Verification items for the finished model (mm, model axes). A direction names the side the tool comes from. Coordinates: 2 decimals unless noted, no trailing zeros. Write each loop counter-clockwise with the first axis right and the second up, starting at its lowest first coordinate (ties: lowest second). Pieces come first, ordered by that corner, then holes. Notation, with made-up numbers: (-38, -1) -> (-18, -1) arc R20 cw to (-18, 33) -> close; hole circle Ø6 at (25.5, 58.25). An arc over 180 degrees is marked (long way). Answer in a Markdown table with one row per item.
```python
from build123d import *

# Parameters (mm, degrees)
F1_DEPTH = 3.302
F2_R     = 3.81
F3_R     = 2.54
F5_D     = 1.905
F6_R     = 1.27


with BuildPart() as f1:
    # F0 (on Top) → F1 (new body)
    with BuildSketch(Plane.XY):
        Polygon((2.54, 0), (0, 0), (0, -18.206947), (-8.938958, -15.811761), (-10.669027, -27.110069), (5.650751, -29.609057), (7.62, -24.926274), (7.62, -14.766274), (3.048, -5.693104), (3.048, -3.547886), (5.588, -3.547886), (5.588, -1.642886), align=None)
    extrude(amount=F1_DEPTH)

    # F2
    f2_edges = [f1.edges().sort_by_distance(p)[0] for p in [
        (0, -18.206947, 1.651),
    ]]
    fillet(f2_edges, radius=F2_R)

    # F3
    f3_edges = [f1.edges().sort_by_distance(p)[0] for p in [
        (-8.938958, -15.811761, 1.651),
    ]]
    fillet(f3_edges, radius=F3_R)

    # F5 (through all)
    with Locations(Plane.XY.offset(3.302)):
        with Locations((6.35, -15.24)):
            Hole(F5_D / 2)

    # F6
    f6_edges = [f1.edges().sort_by_distance(p)[0] for p in [
        (-10.669027, -27.110069, 1.651),
    ]]
    fillet(f6_edges, radius=F6_R)


solid = f1.part
```
1. Go/stop test with flat-tipped pins: pin 1 (1.5 mm diameter, centred on x = 2.5, y = -26.5, fed in from -Z); pin 2 (1.7 mm diameter, centred on y = -4.5, z = 2.5, fed in from +X); pin 3 (1.5 mm diameter, centred on y = -7.5, z = 3, fed in from -X). Record where each tip stops, or that it passes through.
Findings below:
| item | result |
|---|---|
| pin 1 | stops at z = 0 |
| pin 2 | stops at x = 3.05 |
| pin 3 | stops at x = 0 |
2. Material ranges on probe 1 along Y at (x, z) = (5.5, 0.6); probe 2 along X at (y, z) = (-1.75, 2.85); probe 3 along Y at (x, z) = (4.75, 1.8), recorded low to high. Write a range as from..to.
Findings below:
| item | result |
|---|---|
| probe 1 | y = -29.59..-15.67, -14.81..-10.56, -3.55..-1.6 |
| probe 2 | x = 0..5.59 |
| probe 3 | y = -29.47..-9.07, -3.55..-1.19 |
3. Release check for a two-part mould opening along X. For faces 1 (the face through (0, -18, 0)), 2 (the face through (6.62, -27.3, 1.63)), 3 (the face through (-9.915, -22.184, 1.628)), 4 (the face through (-5.488, -16.736, 1.628)) record: released by +X, released by -X, zero draft, split by the parting line, or undercut.
Findings below:
| item | result |
|---|---|
| face 1 | zero draft |
| face 2 | released by +X |
| face 3 | released by -X |
| face 4 | undercut |
4. Sectioned sample at B-B, the plane x = 6.35. Record the cut outline in (y, z).
Findings below:
| item | result |
|---|---|
| outline | (-27.95, 0) -> (-16.19, 0) -> (-16.19, 3.3) -> (-27.95, 3.3) -> close; (-14.29, 0) -> (-12.25, 0) -> (-12.25, 3.3) -> (-14.29, 3.3) -> close |
5. Sectioned sample at D-D, the plane y = -2.75. Record the cut outline in (x, z), and give its area (3 significant figures).
Findings below:
| item | result |
|---|---|
| outline | (0, 0) -> (5.59, 0) -> (5.59, 3.3) -> (0, 3.3) -> close |
| area | 18.5 mm² |
6. Sectioned sample at C-C, the plane y = -15.24. Record the cut outline in (x, z).
Findings below:
| item | result |
|---|---|
| outline | (-0.57, 0) -> (5.4, 0) -> (5.4, 3.3) -> (-0.57, 3.3) -> close; (7.3, 0) -> (7.62, 0) -> (7.62, 3.3) -> (7.3, 3.3) -> close |
7. Access from +Z, -Z, +X, -X, +Y, -Y to the whole of each face (thin tool, end or side, straight path). Record for faces 5 (the face through (5.588, -3, 2)), 6 (the face through (5.366, -10.293, 1.628)), 7 (the face through (0, -18, 3.302)), 8 (the face through (-1.452, -16.234, 1.674)), 9 (the face through (0, -7, 2)).
Findings below:
| item | result |
|---|---|
| face 5 | +Z, -Z, +X, +Y |
| face 6 | +Z, -Z, +X |
| face 7 | +Z, +X, -X, +Y, -Y |
| face 8 | +Z, -Z, +Y |
| face 9 | +Z, -Z, -X, +Y |
